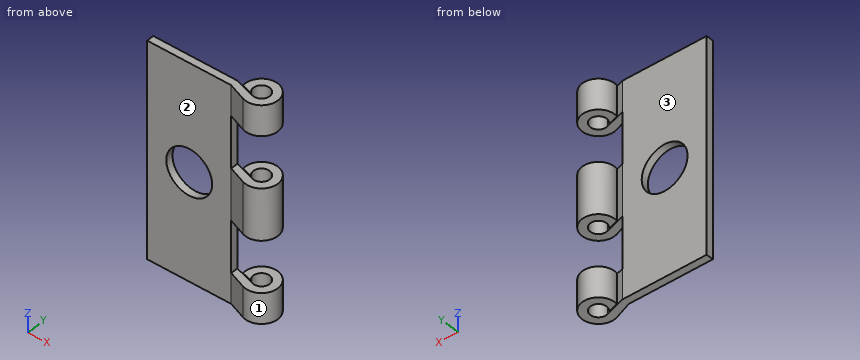
from build123d import *

# Parameters (mm, degrees)
BOSS_EXTRUDE1_DEPTH = 88.9
SKETCH2_W           = 16.271875
SKETCH2_H           = 21.2598
CUT_EXTRUDE1_DEPTH  = 44.45
SKETCH3_R           = 9.525
CUT_EXTRUDE2_DEPTH  = 88.9


with BuildPart() as part:
    # Sketch1 → Boss-Extrude1 (new body)
    with BuildSketch(Plane.XY):
        with BuildLine():
            Line((9.3265625, -3.6068), (16.461695383, -6.309426078))
            ThreePointArc((16.461695383, -6.309426078), (24.035016902, 4.318810338), (12.214407069, -1.21181271))
            Line((12.214407069, -1.21181271), (16.702709255, -2.600482704))
            ThreePointArc((16.702709255, -2.600482704), (20.455010949, 2.968001624), (17.854463061, -3.222712099))
            Line((17.854463061, -3.222712099), (9.3265625, -0.5842))
            Line((9.3265625, -0.5842), (-25.5984375, -0.5842))
            Line((-25.5984375, -0.5842), (-25.5984375, -3.6068))
            Line((-25.5984375, -3.6068), (9.3265625, -3.6068))
        make_face()
    extrude(amount=BOSS_EXTRUDE1_DEPTH)

    # Sketch2 → Cut-Extrude1 (cut, symmetric)
    with BuildSketch(Plane(origin=(0, -0.5842, 0), x_dir=(1, 0, 0), z_dir=(0, 1, 0))):
        with Locations((17.4625, -65.7098)):
            Rectangle(SKETCH2_W, SKETCH2_H)
        with Locations((17.4625, -23.1902)):
            Rectangle(SKETCH2_W, SKETCH2_H)
    extrude(amount=CUT_EXTRUDE1_DEPTH, both=True, mode=Mode.SUBTRACT)

    # Sketch3 → Cut-Extrude2 (cut)
    with BuildSketch(Plane.XZ.offset(3.6068)):
        with Locations((-8.1359375, 44.45)):
            Circle(SKETCH3_R)
    extrude(amount=-CUT_EXTRUDE2_DEPTH, mode=Mode.SUBTRACT)


solid = part.part
Can you work these out from the model? Positions are in its coordinate system, mm. Face numbers are marked on the shaded views. A direction names the side the tool comes from. Give positions to 0.01 mm unless a question says otherwise; leave off trailing zeros. Order: outer loops, then holes, each group sorted by start corner. A loop starts at its lowest first (then second) coordinate and runs counter-clockwise, first axis right, second up. Notation, with made-up numbers: M 64.25,15 L 116.25,15 A26 ccw 116.25,38 Z; hole C 43,57.25 d8. An arc over 180 degrees is marked long. One line per question, with ' | ' between items.
Item 1: Suppose I cut it at B-B, the plane z = 44.45. Write out the boundary of the cut face in (x, y).
Answer block:
outline: M -25.6,-3.61 L -17.66,-3.61 L -17.66,-0.58 L -25.6,-0.58 Z; M 1.39,-3.61 L 9.33,-3.61 L 16.46,-6.31 A6.75 ccw long 12.21,-1.21 L 16.7,-2.6 A3.37 cw long 17.85,-3.22 L 9.33,-0.58 L 1.39,-0.58 Z
Item 2: Suppose I cut it at D-D, the plane x = 10.5. Write out the boundary of the cut face in (y, z).
Answer block:
outline: M -4.05,0 L -0.95,0 L -0.95,12.56 L -4.05,12.56 Z; M -4.05,33.82 L -0.95,33.82 L -0.95,55.08 L -4.05,55.08 Z; M -4.05,76.34 L -0.95,76.34 L -0.95,88.9 L -4.05,88.9 Z
Item 3: I'm going to push flat-ended pins straight in: pin 1 Ø1.5 at (x, z) = (-1, 60) entering from -Y; pin 2 Ø6 at (y, z) = (1.5, 44.5) entering from -X; pin 3 Ø3 at (y, z) = (-3, 42) entering from +X; pin 4 Ø1.5 at (y, z) = (2, 41) entering from -X. Where does each tip first touch, or does it pass through?
Answer block:
pin 1: stops at y = -3.61 | pin 2: stops at x = -25.6 | pin 3: stops at x = 25.43 | pin 4: stops at x = 12.22
Item 4: For the marked faces 1, 2 and 3, which set-ups out of +Z, -Z, +X, -X, +Y, -Y let a thin tool reach every point of the face, with its end or its side?
Answer block:
face 1: +Z, -Z | face 2: +Z, -Z, -X, -Y | face 3: +Z, -Z, -X, +Y
Item 5: Suppose I cut it at A-A, the plane x = 0.5. Write out the boundary of the cut face in (y, z), then the cut area to 3 significant figures.
Answer block:
outline: M -3.61,0 L -0.58,0 L -0.58,40.43 L -3.61,40.43 Z; M -3.61,48.47 L -0.58,48.47 L -0.58,88.9 L -3.61,88.9 Z | area: 244 mm2
Item 6: Please list where these lines run through material, in increasing order: L1, parallel to Z at x = 17.5, y = 5.5; L2, parallel to X at y = 0, z = 8 (3 decimals); L3, parallel to X at y = -2.5, z = 59.
Answer block:
L1: z = 0 to 12.56, 33.82 to 55.08, 76.34 to 88.9 | L2: x = 12.105 to 15.478, 22.225 to 25.598 | L3: x = -25.6 to 9.33
Item 7: Suppose I cut it at C-C, the plane y = 4.5. Write out the boundary of the cut face in (x, z), then the cut area to 3 significant figures.
Answer block:
outline: M 13.82,0 L 23.88,0 L 23.88,12.56 L 13.82,12.56 Z; M 13.82,33.82 L 23.88,33.82 L 23.88,55.08 L 13.82,55.08 Z; M 13.82,76.34 L 23.88,76.34 L 23.88,88.9 L 13.82,88.9 Z | area: 466 mm2
